from build123d import *

# Parameters (mm, degrees)
SKETCH1_R               = 184.15
BOSS_EXTRUDE1_DEPTH     = 2.54
CUT_EXTRUDE1_DEPTH      = 261.439813777
CUT_EXTRUDE1_DEPTH_BACK = 261.439813777


with BuildPart() as part:
    # Sketch1 → Boss-Extrude1 (new body)
    with BuildSketch(Plane.XY):
        Circle(SKETCH1_R)
    extrude(amount=BOSS_EXTRUDE1_DEPTH)

    # Sketch2 → Cut-Extrude1 (cut, two sides: drawn at the far end of the back side and taken through both)
    with BuildSketch(Plane.XY.offset(2.54).offset(-CUT_EXTRUDE1_DEPTH_BACK)):
        with BuildLine():
            Line((-105.302837094, -44.45), (-152.4, -44.45))
            ThreePointArc((-152.4, -44.45), (-159.026348403, 0), (-152.4, 44.45))
            Line((-152.4, 44.45), (-105.302837094, 44.45))
            ThreePointArc((-105.302837094, 44.45), (114.3, 0), (-105.302837094, -44.45))
        make_face()
    extrude(amount=CUT_EXTRUDE1_DEPTH + CUT_EXTRUDE1_DEPTH_BACK, mode=Mode.SUBTRACT)


solid = part.part
The model under review builds one solid part; all positions refer to its coordinate system, in mm. Give positions to 0.01 mm unless a question says otherwise; leave off trailing zeros. Write each loop counter-clockwise with the first axis right and the second up, starting at its lowest first coordinate (ties: lowest second). Pieces come first, ordered by that corner, then holes.
1. Add section C-C, the plane z = 1.6. Write out the cut boundary in (x, y), plus the area to 3 significant figures.
2. Add section D-D, the plane y = -150. Write out the cut boundary in (x, z).
3. Add section A-A, the plane x = 0. Write out the cut boundary in (y, z).
4. Draft analysis for pull direction X (two halves, no side actions). For faces 1 (the cylindrical face through (114.216, 4.387, 1.252)), 2 (the cylindrical face through (-146.1, -112.1, 1.3)), 3 (the flat face through (120, 3, 0)), state which applies: +X half, -X half, draft (parallel to the pull), parting line (faces both ways), or undercut.
5. Add section B-B, the plane y = 0. Write out the cut boundary in (x, z).
6. For P1, Ø1.5, axis at x = -142, z = 2, coming from the +Y side; P2, Ø0.8, axis at x = -139, z = 0.5, coming from the +Y side; P3, Ø1, axis at y = -77.5, z = 2, coming from the +X side, all flat-tipped, find the tip position at first contact; note any pin that passes through.
7. Wall thickness on L1, parallel to Y at x = 0, z = 0.5; L2, parallel to X at y = -1, z = 1.7; L3, parallel to Y at x = -60.5, z = 2.1: over which ranges is each line inside the solid? List them lowest first.
Worked answers:
1. outline: circle Ø368.3 at (0, 0); hole (-152.4, -44.45) - (-105.3, -44.45) arc R114.3 ccw (long way) to (-105.3, 44.45) - (-152.4, 44.45) arc R152.4 ccw to start
1. area: 61,400 mm2
2. outline: (-106.82, 0) - (106.82, 0) - (106.82, 2.54) - (-106.82, 2.54) - close
3. outline: (-184.15, 0) - (-114.3, 0) - (-114.3, 2.54) - (-184.15, 2.54) - close; (114.3, 0) - (184.15, 0) - (184.15, 2.54) - (114.3, 2.54) - close
4. face 1: undercut
4. face 2: parting line
4. face 3: draft
5. outline: (-184.15, 0) - (-159.03, 0) - (-159.03, 2.54) - (-184.15, 2.54) - close; (114.3, 0) - (184.15, 0) - (184.15, 2.54) - (114.3, 2.54) - close
6. P1: stops at y = 118.15
6. P2: stops at y = 121.25
6. P3: stops at x = 167.28
7. L1: y = -184.15 to -114.3, 114.3 to 184.15
7. L2: x = -184.15 to -159.02, 114.3 to 184.15
7. L3: y = -173.93 to -96.98, 96.98 to 173.93
